Verification items for the finished model (mm, model axes). Face numbers are marked on the shaded views. A direction names the side the tool comes from. Coordinates: 2 decimals unless noted, no trailing zeros. Order: outer loops, then holes, each group sorted by start corner. A loop starts at its lowest first (then second) coordinate and runs counter-clockwise, first axis right, second up. Notation, with made-up numbers: M 55.25,-27.75 L 95.25,-27.75 A17 ccw 95.25,-14.75 Z; hole C 26.5,59 d2. An arc over 180 degrees is marked long. Answer as a JSON object with one key per item and string values. Group by question number.
(1) Cross-section at D-D (x = 17.25). Enter the section's corners in (y, z).
(2) Cross-section at A-A (z = 2). Enter the section's corners in (x, y).
(3) Cross-section at B-B (y = 1.6). Count the separate pieces of the cut face and the enclosed holes in it, plus the area to 3 significant figures.
(4) Material ranges on line 1 (Y direction, x = 4.5, z = 1.6); line 2 (Y direction, x = 17.25, z = 0.85), recorded low to high.
(5) Access from +Z, -Z, +X, -X, +Y, -Y to the whole of each face (thin tool, end or side, straight path). Record for the marked faces 5 and 6.
(6) Cross-section at C-C (x = 1.75). Enter the section's corners in (y, z).
(7) Mould release check, pull along X, two halves, no side actions. Record for the marked faces 1, 2, 3 and 4: released by +X, released by -X, zero draft, split by the parting line, or undercut.
from build123d import *

# Parameters (mm, degrees)
F1_DEPTH = 3


with BuildPart() as f1:
    # F0 (on Top) → F1 (new body)
    with BuildSketch(Plane.XY):
        Polygon((1, 2), (0, 0), (2, 0), align=None)
        Polygon((2, 0), (0, 0), (0, -3.129371), (20, -3.129371), (20, 0), (18, 0), (16, 0), (14, 0), (12, 0), (10, 0), (8, 0), (6, 0), (4, 0), align=None)
        Polygon((3, 2), (2, 0), (4, 0), align=None)
        Polygon((5, 2), (4, 0), (6, 0), align=None)
        Polygon((7, 2), (6, 0), (8, 0), align=None)
        Polygon((18, 0), (20, 0), (19, 2), align=None)
        Polygon((9, 2), (8, 0), (10, 0), align=None)
        Polygon((16, 0), (18, 0), (17, 2), align=None)
        Polygon((11, 2), (10, 0), (12, 0), align=None)
        Polygon((14, 0), (16, 0), (15, 2), align=None)
        Polygon((13, 2), (12, 0), (14, 0), align=None)
    extrude(amount=F1_DEPTH)


solid = f1.part
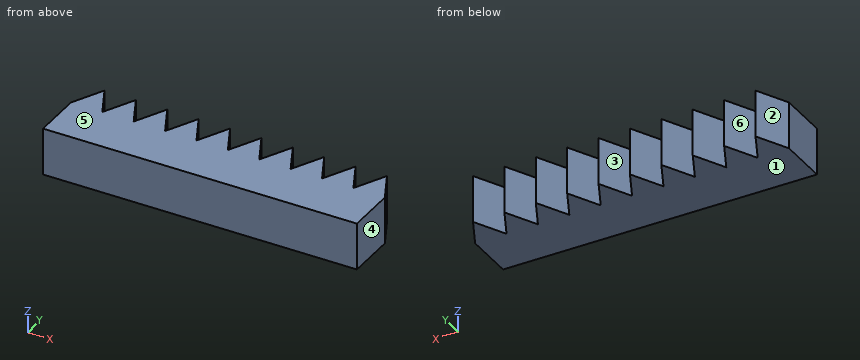
Taken from the geometry:
{
 "1": {"outline": "M -3.13,0 L 1.5,0 L 1.5,3 L -3.13,3 Z"},
 "2": {"outline": "M 0,-3.13 L 20,-3.13 L 20,0 L 19,2 L 18,0 L 17,2 L 16,0 L 15,2 L 14,0 L 13,2 L 12,0 L 11,2 L 10,0 L 9,2 L 8,0 L 7,2 L 6,0 L 5,2 L 4,0 L 3,2 L 2,0 L 1,2 L 0,0 Z"},
 "3": {"separate pieces": "10", "enclosed holes": "0", "area": "12.0 mm²"},
 "4": {"line 1": "y = -3.13 to 1", "line 2": "y = -3.13 to 1.5"},
 "5": {"face 5": "+Z, +X, -X, +Y, -Y", "face 6": "+Z, -Z, +Y"},
 "6": {"outline": "M -3.13,0 L 0.5,0 L 0.5,3 L -3.13,3 Z"},
 "7": {"face 1": "zero draft", "face 2": "released by -X", "face 3": "undercut", "face 4": "released by +X"}
}
